Model file for the job. Use its own axes, mm. Face numbers are marked on the shaded views. A direction names the side the tool comes from. Coordinates: 2 decimals unless noted, no trailing zeros. Order: outer loops, then holes, each group sorted by start corner. A loop starts at its lowest first (then second) coordinate and runs counter-clockwise, first axis right, second up. Notation, with made-up numbers: (-30.5, 46) - (-4.5, 46) arc R7 cw to (-4.5, 59) - close; hole circle Ø5 at (23.5, 34). An arc over 180 degrees is marked (long way). Put each result on its own line as item: value. Start each with the question number.
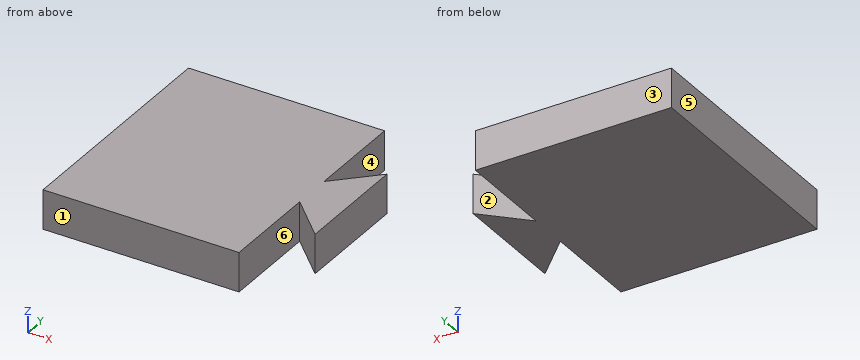
```python
from build123d import *

# Parameters (mm, degrees)
SKETCH_2_W      = 50
SKETCH_2_H      = 60
EXTRUDE_1_DEPTH = 10
SKETCH_4_W      = 10
SKETCH_4_H      = 10
EXTRUDE_2_DEPTH = 10
EXTRUDE_3_DEPTH = 10


with BuildPart() as part:
    # 草图2 → 凸台-拉伸1 (new body)
    with BuildSketch(Plane.XY):
        with Locations((-17.786885246, -14.016393443)):
            Rectangle(SKETCH_2_W, SKETCH_2_H)
    extrude(amount=EXTRUDE_1_DEPTH)

    # 草图4 → 凸台-拉伸2 (add)
    with BuildSketch(Plane.XY.offset(10)):
        with Locations((12.213114754, -14.016393443)):
            Rectangle(SKETCH_4_W, SKETCH_4_H)
    extrude(amount=-EXTRUDE_2_DEPTH)

    # 草图5 → 凸台-拉伸3 (add)
    with BuildSketch(Plane.XY.offset(10)):
        Polygon((7.213114754, -9.016393443), (17.213114754, 0.810579189), (17.213114754, -9.016393443), align=None)
        Polygon((7.213114754, -19.016393443), (17.213114754, -19.016393443), (17.213114754, -28.843366074), align=None)
    extrude(amount=-EXTRUDE_3_DEPTH)


solid = part.part
```
Item 1: 3-axis set-ups, long thin cutter, end or side, ignore diameter. For the marked faces 1 and 2: which of +Z, -Z, +X, -X, +Y, -Y reach the whole face in a straight line?
Item 2: Slice it at C-C, the plane y = -1. Give the cut face in (x, z).
Item 3: Wall check: line 1 along X through (y, z) = (-35.5, 1.5); line 2 along X through (y, z) = (-22, 7); line 3 along X through (y, z) = (-21, 6.5). Give the ranges that are in metal, low to high.
Item 4: Slice it at A-A, the plane y = -27. Give the cut face in (x, z), plus the area to 3 significant figures.
Item 5: Slice it at D-D, the plane x = 9. Give the cut face in (y, z).
Item 6: Pull direction X, two halves, no side cores. Call the marked faces 3, 4, 5 and 6: pulls with the +X half, pulls with the -X half, needs draft (parallel to the pull), parting line crosses it, or undercut.
Item 7: Slice it at B-B, the plane z = 1.25. Give the cut face in (x, y), plus the area to 3 significant figures.
Here are the results:
1. face 1: +Z, -Z, +X, -X, -Y
1. face 2: +Z, -Z, +Y
2. outline: (-42.79, 0) - (7.21, 0) - (7.21, 10) - (-42.79, 10) - close; (15.37, 0) - (17.21, 0) - (17.21, 10) - (15.37, 10) - close
3. line 1: x = -42.79 to 7.21
3. line 2: x = -42.79 to 7.21, 10.25 to 17.21
3. line 3: x = -42.79 to 7.21, 9.23 to 17.21
4. outline: (-42.79, 0) - (7.21, 0) - (7.21, 10) - (-42.79, 10) - close; (15.34, 0) - (17.21, 0) - (17.21, 10) - (15.34, 10) - close
4. area: 519 mm^2
5. outline: (-20.77, 0) - (-7.26, 0) - (-7.26, 10) - (-20.77, 10) - close
6. face 3: needs draft
6. face 4: undercut
6. face 5: pulls with the -X half
6. face 6: undercut
7. outline: (-42.79, -44.02) - (7.21, -44.02) - (7.21, -19.02) - (17.21, -28.84) - (17.21, 0.81) - (7.21, -9.02) - (7.21, 15.98) - (-42.79, 15.98) - close
7. area: 3,200 mm^2
